Can you work these out from the drawing? Everything is in mm from the part's minimum corner. A direction names the side the tool comes from. Coordinates: 2 decimals unless noted, no trailing zeros. Loops run counter-clockwise (first coordinate to the right, second up) from the corner with the lowest first, then second, coordinate; pieces in that order, holes last.
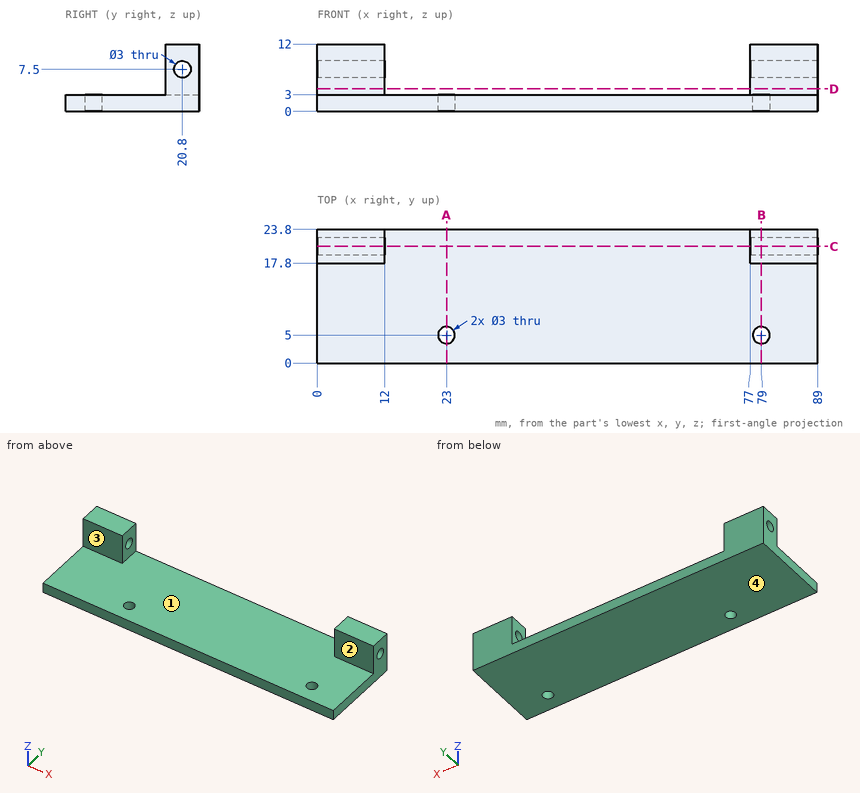
Item 1: Suppose I cut it at B-B, the plane x = 79. Please give me the cut outline in (y, z).
Results are:
outline: (0, 0) - (3.5, 0) - (3.5, 3) - (0, 3) - close; (6.5, 0) - (23.8, 0) - (23.8, 12) - (17.8, 12) - (17.8, 3) - (6.5, 3) - close; hole circle Ø3 at (20.8, 7.5)
Item 2: On a 3-axis mill with a long thin cutter (end or side, diameter ignored), from which of +Z, -Z, +X, -X, +Y, -Y can I reach the whole of each face in a straight line? I mean the marked faces 3 and 4. Say none if no direction works.
Results are:
face 3: +Z, +X, -X, -Y
face 4: -Z, +X, -X, +Y, -Y
Item 3: Suppose I cut it at A-A, the plane x = 23. Please give me the cut outline in (y, z), plus the area to 3 significant figures.
Results are:
outline: (0, 0) - (3.5, 0) - (3.5, 3) - (0, 3) - close; (6.5, 0) - (23.8, 0) - (23.8, 3) - (6.5, 3) - close
area: 62.4 mm2
Item 4: We'd pull the mould along X, two halves only. Please class the marked faces 1 and 2: +X half, -X half, draft (parallel to the pull), parting line (faces both ways), or undercut.
Results are:
face 1: undercut
face 2: draft
Item 5: I need wall thicknesses on line 1 along Z through (x, y) = (81.75, 20.8); line 2 along Y through (x, z) = (79, 2.2); line 3 along X through (y, z) = (21.25, 5.25). Which ranges of each line are inside material? Lowest first, please.
Results are:
line 1: z = 0 to 6, 9 to 12
line 2: y = 0 to 3.5, 6.5 to 23.8
line 3: x = 0 to 12, 77 to 89
Item 6: Suppose I cut it at C-C, the plane y = 20.8. Please give me the cut outline in (x, z).
Results are:
outline: (0, 0) - (89, 0) - (89, 6) - (77, 6) - (77, 3) - (12, 3) - (12, 6) - (0, 6) - close; (0, 9) - (12, 9) - (12, 12) - (0, 12) - close; (77, 9) - (89, 9) - (89, 12) - (77, 12) - close
Item 7: I'm going to push flat-ended pins straight in: P1, Ø4, axis at x = 23, y = 5, coming from the +Z side; P2, Ø2.5, axis at x = 85, z = 8.5, coming from the -Y side. Where does each tip first touch, or does it pass through?
Results are:
P1: stops at z = 3
P2: stops at y = 17.8
Item 8: Suppose I cut it at D-D, the plane z = 4. Please give me the cut outline in (x, y), plus the area to 3 significant figures.
Results are:
outline: (0, 17.8) - (12, 17.8) - (12, 23.8) - (0, 23.8) - close; (77, 17.8) - (89, 17.8) - (89, 23.8) - (77, 23.8) - close
area: 144 mm2
